from build123d import *

# Parameters (mm, degrees)
BOSS_EXTRUDE1_DEPTH = 1
BOSS_EXTRUDE2_START = -6
BOSS_EXTRUDE2_DEPTH = 6
SKETCH4_R           = 33.5
SKETCH4_R_2         = 32.5
BOSS_EXTRUDE3_DEPTH = 26
CUT_EXTRUDE3_START  = -1
SKETCH4_4_R         = 32.5
CUT_EXTRUDE3_DEPTH  = 27
FILLET2_R           = 1


with BuildPart() as part:
    # Sketch1 → Boss-Extrude1 (new body)
    with BuildSketch(Plane(origin=(0, 0, 0), x_dir=(1, 0, 0), z_dir=(0, 1, 0))):
        with BuildLine():
            Line((121, 23), (121, 87))
            Line((121, 87), (0, 87))
            ThreePointArc((0, 87), (-54.254032108, -68.011028517), (84.824655745, 19.333333333))
            ThreePointArc((84.824655745, 19.333333333), (85.404435994, 21.870828693), (87.749643874, 23))
            Line((87.749643874, 23), (121, 23))
        make_face()
    extrude(amount=BOSS_EXTRUDE1_DEPTH)

    # Sketch1<3> → Boss-Extrude2 (add)
    with BuildSketch(Plane(origin=(0, 0, 0), x_dir=(1, 0, 0), z_dir=(0, 1, 0)).offset(BOSS_EXTRUDE2_START)):
        with BuildLine():
            Line((121, 23), (121, 24))
            Line((121, 24), (87.749643874, 24))
            ThreePointArc((87.749643874, 24), (84.622700034, 22.494438258), (83.849659702, 19.111111111))
            ThreePointArc((83.849659702, 19.111111111), (-53.630422544, -67.229292557), (0, 86))
            Line((0, 86), (121, 86))
            Line((121, 86), (121, 87))
            Line((121, 87), (0, 87))
            ThreePointArc((0, 87), (-54.254032108, -68.011028517), (84.824655745, 19.333333333))
            ThreePointArc((84.824655745, 19.333333333), (85.404435994, 21.870828693), (87.749643874, 23))
            Line((87.749643874, 23), (121, 23))
        make_face()
    extrude(amount=BOSS_EXTRUDE2_DEPTH)

    # Sketch4 → Boss-Extrude3 (add)
    # profile 1 of 2: a face of its own
    with BuildSketch(Plane(origin=(0, 1, 0), x_dir=(1, 0, 0), z_dir=(0, 1, 0))):
        with Locations(Location((0, 0, 0), (0, 0, 90))):
            Circle(SKETCH4_R)
        Circle(SKETCH4_R_2, mode=Mode.SUBTRACT)
    # profile 2 of 2: a face of its own
    with BuildSketch(Plane(origin=(0, 1, 0), x_dir=(1, 0, 0), z_dir=(0, 1, 0))):
        Circle(SKETCH4_R_2)
    extrude(amount=BOSS_EXTRUDE3_DEPTH)

    # Sketch4<4> → Cut-Extrude3 (cut)
    with BuildSketch(Plane(origin=(0, 1, 0), x_dir=(1, 0, 0), z_dir=(0, 1, 0)).offset(CUT_EXTRUDE3_START)):
        with Locations(Location((0, 0, 0), (0, 0, 270))):
            Circle(SKETCH4_4_R)
    extrude(amount=CUT_EXTRUDE3_DEPTH, mode=Mode.SUBTRACT)

    # Fillet2
    fillet2_edges = [part.edges().sort_by_distance(p)[0] for p in [
        (60.5, 1, -87),
        (-54.254032108, 1, 68.011028517),
        (-53.630422544, 0, 67.229292557),
        (85.404435994, 1, -21.870828693),
        (104.374821937, 0, -24),
        (84.622700034, 0, -22.494438258),
        (60.5, 0, -86),
        (104.374821937, 1, -23),
        (0, 1, 33.5),
        (0, 27, 33.5),
        (0, 0, -32.5),
    ]]
    fillet(fillet2_edges, radius=FILLET2_R - 0.0001)  # a hair under: the kernel refuses the full size


solid = part.part
The model under review builds one solid part; all positions refer to its coordinate system, in mm. A direction names the side the tool comes from. Coordinates: 2 decimals unless noted, no trailing zeros. Loops run counter-clockwise (first coordinate to the right, second up) from the corner with the lowest first, then second, coordinate; pieces in that order, holes last. Notation, with made-up numbers: (64, 14) -> (116, 14) arc R23 ccw to (116, 42) -> close; hole circle Ø4 at (-6.5, 62). An arc over 180 degrees is marked (long way). Use a Markdown table: item, result. Add a question column.
1. Draft analysis for pull direction X (two halves, no side actions). For faces 6 (the face through (60, -4, -86)), 7 (the face through (-51.28, -3.53, 69.04)), 8 (the face through (-56.571, -3.042, 66.096)), state which applies: pulls with the +X half, pulls with the -X half, needs draft (parallel to the pull), parting line crosses it, or undercut.
2. Clearance check with flat-ended pins moving along their axes: pin 1 Ø8 at (x, z) = (86, 18.5) entering from +Y; pin 2 Ø3 at (x, y) = (110.5, -2) entering from +Z; pin 3 Ø12 at (y, z) = (20.5, 14) entering from +X. State where each tip first meets the part, or that it passes through.
3. Add section A-A on y = 20. Write out the cut boundary in (x, z).
4. Machinability: for faces 1 (the face through (121, 0.3, -54.9)), 2 (the face through (104, -3, -23)), 3 (the face through (84.65, -3.53, -22.53)), 4 (the face through (39, 1, -1)), 5 (the face through (105, -4, -24)), which of the approach directions +Z, -Z, +X, -X, +Y, -Y give a long, thin tool a straight path to every point of the face, cutting with its end or side? Answer none if there is none.
5. To check wall thickness, follow line 1 (Z direction, x = 0, y = -4.35); line 2 (X direction, y = 11, z = 0). State the ranges of each line that lie inside material, in increasing order.
Returned:
| question | item | result |
|---|---|---|
| 1 | face 6 | needs draft |
| 1 | face 7 | undercut |
| 1 | face 8 | parting line crosses it |
| 2 | pin 1 | stops at y = 1 |
| 2 | pin 2 | stops at z = -23 |
| 2 | pin 3 | stops at x = 32.53 |
| 3 | outline | circle Ø67 at (0, 0); hole circle Ø65 at (0, 0) |
| 4 | face 1 | +Z, -Z, +X, +Y, -Y |
| 4 | face 2 | +Z, +X, +Y, -Y |
| 4 | face 3 | -Y |
| 4 | face 4 | +Y |
| 4 | face 5 | +X, -Y |
| 5 | line 1 | z = -87 to -86, 86 to 87 |
| 5 | line 2 | x = -33.5 to -32.5, 32.5 to 33.5 |
